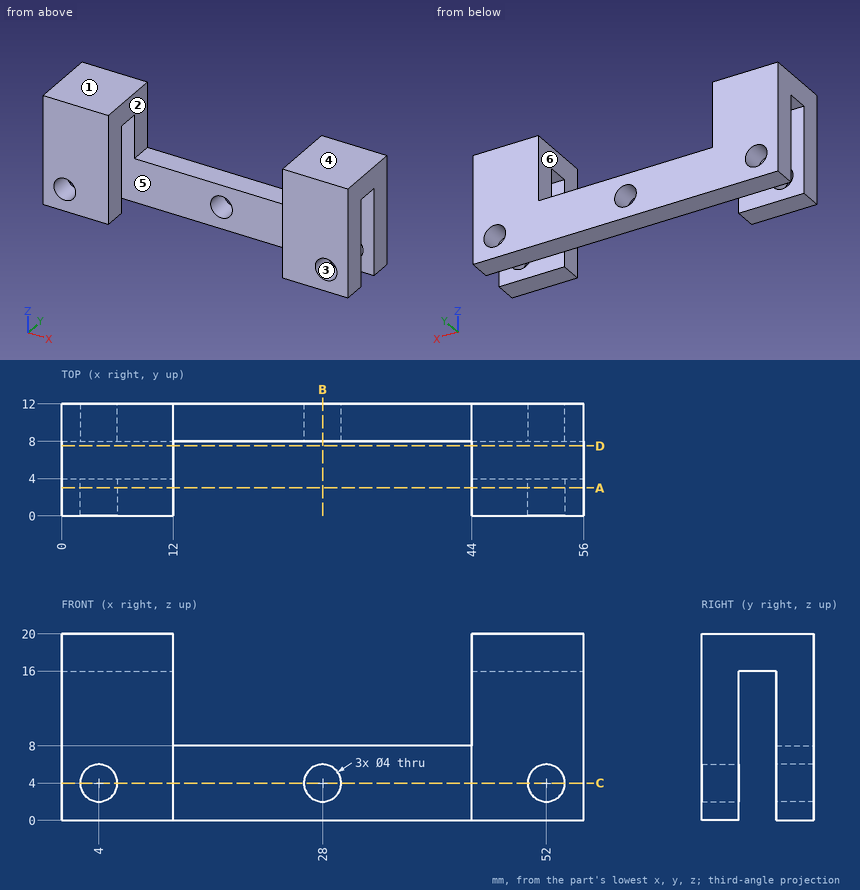
For this review, use the dimensioned drawing (mm, ordinates from the lowest corner) and the shaded views. A direction names the side the tool comes from. Give positions to 0.01 mm unless a question says otherwise; leave off trailing zeros. Order: outer loops, then holes, each group sorted by start corner. A loop starts at its lowest first (then second) coordinate and runs counter-clockwise, first axis right, second up.
1. Add section C-C, the plane z = 4. State how many separate pieces and enclosed holes the cut face has, then the cut area to 3 significant figures.
Solution:
separate pieces: 8
enclosed holes: 0
area: 240 mm2
2. Tool access review of the marked faces 4, 5 and 6: name each direction out of +Z, -Z, +X, -X, +Y, -Y from which nothing blocks a thin tool from reaching the whole face with its end or side.
Solution:
face 4: +Z, +X, -X, +Y, -Y
face 5: -Z, +X, -X
face 6: +Z, -Y
3. Add section B-B, the plane x = 28. State the section outline as (y, z) points.
Solution:
outline: (8, 0) - (12, 0) - (12, 2) - (8, 2) - close; (8, 6) - (12, 6) - (12, 8) - (8, 8) - close
4. Mouldability with a two-part tool opening along Z and no side actions: class the marked faces 1, 2 and 3 as +Z half, -Z half, draft (parallel to the pull), parting line (faces both ways), or undercut.
Solution:
face 1: +Z half
face 2: draft
face 3: undercut
5. For pin 1 Ø1 at (x, z) = (42, 6.5) entering from -Y; pin 2 Ø4.5 at (x, y) = (27, 9.5) entering from +Z; pin 3 Ø1.2 at (x, y) = (5.5, 6) entering from -Z, all flat-tipped, find the tip position at first contact; note any pin that passes through.
Solution:
pin 1: stops at y = 8
pin 2: stops at z = 8
pin 3: stops at z = 16
6. Add section A-A, the plane y = 3. State the section outline as (x, z) points, then the cut area to 3 significant figures.
Solution:
outline: (0, 0) - (12, 0) - (12, 20) - (0, 20) - close; (44, 0) - (56, 0) - (56, 20) - (44, 20) - close; hole circle Ø4 at (4, 4); hole circle Ø4 at (52, 4)
area: 455 mm2
7. Add section D-D, the plane y = 7.5. State the section outline as (x, z) points, then the cut area to 3 significant figures.
Solution:
outline: (0, 16) - (12, 16) - (12, 20) - (0, 20) - close; (44, 16) - (56, 16) - (56, 20) - (44, 20) - close
area: 96.0 mm2
8. To check wall thickness, follow L1, parallel to X at y = 9.5, z = 18.75; L2, parallel to X at y = 11.25, z = 3; L3, parallel to Z at x = 28, y = 10.05. State the ranges of each line that lie inside material, in increasing order.
Solution:
L1: x = 0 to 12, 44 to 56
L2: x = 0 to 2.27, 5.73 to 26.27, 29.73 to 50.27, 53.73 to 56
L3: z = 0 to 2, 6 to 8
